Source: CAD feature listing. Evaluate the final solid. Frame: model axes, mm. A direction names the side the tool comes from. Round coordinates to 2 decimals unless told otherwise and drop trailing zeros. Loops run counter-clockwise (first coordinate to the right, second up) from the corner with the lowest first, then second, coordinate; pieces in that order, holes last. Notation, with made-up numbers: M 27.5,71 L 53.5,71 A27 ccw 53.5,92 Z; hole C 33,34.5 d11. An arc over 180 degrees is marked long. One line per item, written item: value.
from build123d import *

# Parameters (mm, degrees)
SKETCH2_R          = 2.5
CUT_EXTRUDE1_DEPTH = 23.045407685


with BuildPart() as part:
    # Sketch1 → Revolve1 (revolve)
    with BuildSketch(Plane.XY, mode=Mode.PRIVATE) as revolve1_sk:
        Polygon((0, 0), (0, 5), (2, 5), (2, 9), (4, 9), (4, 5), (14, 5), (14, 9), (16, 9), (16, 5), (18, 5), (18, 0), align=None)
    revolve(revolve1_sk.sketch.rotate(Axis((0, 0, 0), (1, 0, 0)), 90), axis=Axis((0, 0, 0), (1, 0, 0)))

    # Sketch2 → Cut-Extrude1 (cut, through all)
    with BuildSketch(Plane(origin=(18, 0, 0), x_dir=(0, 0, -1), z_dir=(1, 0, 0))):
        Circle(SKETCH2_R)
    extrude(amount=-CUT_EXTRUDE1_DEPTH, mode=Mode.SUBTRACT)


solid = part.part
1. Pin query (flat end, axial travel): pin 1 (2 mm diameter, centred on y = -3, z = -6.5, fed in from -X); pin 2 (10 mm diameter, centred on x = 16, y = -6.5, fed in from +Z); pin 3 (1 mm diameter, centred on x = 3.5, y = 3.5, fed in from -Z); pin 4 (6 mm diameter, centred on x = 4, y = 2.5, fed in from +Z). Return the tip coordinate at first contact, or that it passes through.
Report:
pin 1: stops at x = 2
pin 2: stops at z = 8.87
pin 3: stops at z = -8.49
pin 4: stops at z = 9
2. Ray query, line 1 (X direction, y = 5, z = 2); line 2 (Y direction, x = 8.25, z = 0); line 3 (Y direction, x = 13.5, z = -1.25). Return the intervals inside material, ascending. Write a range as [from, to].
Report:
line 1: x = [2, 4], [14, 16]
line 2: y = [-5, -2.5], [2.5, 5]
line 3: y = [-4.84, -2.17], [2.17, 4.84]
3. Section query C-C (x = 16.5). Return the cut outline in (y, z), and give its area (3 significant figures).
Report:
outline: C 0,0 d10; hole C 0,0 d5
area: 58.9 mm2
4. Pull-direction query (Y, two-part tool) for faces 6 (the face through (16, 4, 4)), 7 (the face through (9.13, -2.44, 0.54)), 8 (the face through (3.014, -6.083, -6.633)); classes: released by +Y, released by -Y, zero draft, split by the parting line, or undercut.
Report:
face 6: zero draft
face 7: undercut
face 8: split by the parting line
5. Reachability of faces 1 (the face through (0, 2, -2)), 2 (the face through (2, 4, -4)), 3 (the face through (18, 2, 2)), 4 (the face through (17, 0, -5)), 5 (the face through (4, 4, 4)) from +Z, -Z, +X, -X, +Y, -Y: full face, straight path, thin tool, end or side. Return the list, or none.
Report:
face 1: +Z, -Z, -X, +Y, -Y
face 2: -X
face 3: +Z, -Z, +X, +Y, -Y
face 4: +X
face 5: none
6. Section query A-A (y = 0). Return the cut outline in (x, z), and give its area (3 significant figures).
Report:
outline: M 0,-5 L 2,-5 L 2,-9 L 4,-9 L 4,-5 L 14,-5 L 14,-9 L 16,-9 L 16,-5 L 18,-5 L 18,-2.5 L 0,-2.5 Z; M 0,2.5 L 18,2.5 L 18,5 L 16,5 L 16,9 L 14,9 L 14,5 L 4,5 L 4,9 L 2,9 L 2,5 L 0,5 Z
area: 122 mm2
7. Section query D-D (y = 4). Return the cut outline in (x, z), and give its area (3 significant figures).
Report:
outline: M 0,-3 L 2,-3 L 2,-8.06 L 4,-8.06 L 4,-3 L 14,-3 L 14,-8.06 L 16,-8.06 L 16,-3 L 18,-3 L 18,3 L 16,3 L 16,8.06 L 14,8.06 L 14,3 L 4,3 L 4,8.06 L 2,8.06 L 2,3 L 0,3 Z
area: 148 mm2
